Model file for the job. Use its own axes, mm. Face numbers are marked on the shaded views. A direction names the side the tool comes from. Coordinates: 2 decimals unless noted, no trailing zeros. Order: outer loops, then holes, each group sorted by start corner. A loop starts at its lowest first (then second) coordinate and runs counter-clockwise, first axis right, second up.
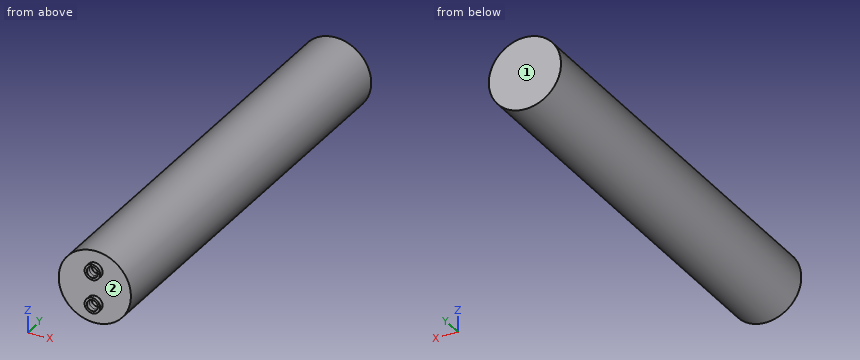
from build123d import *

# Parameters (mm, degrees)
F0_R     = 6.5
F1_DEPTH = 79
F2_T     = -0.8
F3_DEPTH = 0.8
F4_DEPTH = 0.8


with BuildPart() as f1:
    # F0 (on Front) → F1 (new body)
    with BuildSketch(Plane.XZ):
        with Locations((6.5, 6.5)):
            Circle(F0_R)
        with BuildLine():
            ThreePointArc((7.9, 3.5), (5.5100505063, 2.5100505063), (6.5, 4.9))
            ThreePointArc((6.5, 4.9), (7.4899494937, 4.4899494937), (7.9, 3.5))
        make_face(mode=Mode.SUBTRACT)
        with BuildLine():
            ThreePointArc((6.5, 8.1), (5.5100505063, 10.4899494937), (7.9, 9.5))
            ThreePointArc((7.9, 9.5), (7.4899494937, 8.5100505063), (6.5, 8.1))
        make_face(mode=Mode.SUBTRACT)
        with BuildLine():
            ThreePointArc((6.5, 8.1), (7.4899494937, 8.5100505063), (7.9, 9.5))
            ThreePointArc((7.9, 9.5), (5.5100505063, 10.4899494937), (6.5, 8.1))
        make_face()
        with BuildLine():
            ThreePointArc((7.5, 9.5), (7.2071067812, 8.7928932188), (6.5, 8.5))
            ThreePointArc((6.5, 8.5), (5.7928932188, 10.2071067812), (7.5, 9.5))
        make_face(mode=Mode.SUBTRACT)
        with BuildLine():
            ThreePointArc((7.9, 3.5), (7.4899494937, 4.4899494937), (6.5, 4.9))
            ThreePointArc((6.5, 4.9), (5.5100505063, 2.5100505063), (7.9, 3.5))
        make_face()
        with BuildLine():
            ThreePointArc((7.5, 3.5), (5.7928932188, 2.7928932188), (6.5, 4.5))
            ThreePointArc((6.5, 4.5), (7.2071067812, 4.2071067812), (7.5, 3.5))
        make_face(mode=Mode.SUBTRACT)
        with BuildLine():
            ThreePointArc((7.5, 9.5), (5.7928932188, 10.2071067812), (6.5, 8.5))
            ThreePointArc((6.5, 8.5), (7.2071067812, 8.7928932188), (7.5, 9.5))
        make_face()
        with BuildLine():
            ThreePointArc((7.5, 3.5), (7.2071067812, 4.2071067812), (6.5, 4.5))
            ThreePointArc((6.5, 4.5), (5.7928932188, 2.7928932188), (7.5, 3.5))
        make_face()
    extrude(amount=-F1_DEPTH)

    # F2
    f2_openings = [f1.faces().sort_by_distance(p)[0] for p in [
        (6.5, 0, 6.5),
    ]]
    offset(amount=F2_T, openings=f2_openings)

    # F0 (on Front) → F3 (join)
    with BuildSketch(Plane.XZ):
        with Locations((6.5, 6.5)):
            Circle(F0_R)
        with BuildLine():
            ThreePointArc((7.9, 3.5), (5.5100505063, 2.5100505063), (6.5, 4.9))
            ThreePointArc((6.5, 4.9), (7.4899494937, 4.4899494937), (7.9, 3.5))
        make_face(mode=Mode.SUBTRACT)
        with BuildLine():
            ThreePointArc((6.5, 8.1), (5.5100505063, 10.4899494937), (7.9, 9.5))
            ThreePointArc((7.9, 9.5), (7.4899494937, 8.5100505063), (6.5, 8.1))
        make_face(mode=Mode.SUBTRACT)
    extrude(amount=-F3_DEPTH)

    # F0 (on Front) → F4 (join, symmetric)
    with BuildSketch(Plane.XZ):
        with BuildLine():
            ThreePointArc((6.5, 8.1), (7.4899494937, 8.5100505063), (7.9, 9.5))
            ThreePointArc((7.9, 9.5), (5.5100505063, 10.4899494937), (6.5, 8.1))
        make_face()
        with BuildLine():
            ThreePointArc((7.5, 9.5), (7.2071067812, 8.7928932188), (6.5, 8.5))
            ThreePointArc((6.5, 8.5), (5.7928932188, 10.2071067812), (7.5, 9.5))
        make_face(mode=Mode.SUBTRACT)
        with BuildLine():
            ThreePointArc((7.9, 3.5), (7.4899494937, 4.4899494937), (6.5, 4.9))
            ThreePointArc((6.5, 4.9), (5.5100505063, 2.5100505063), (7.9, 3.5))
        make_face()
        with BuildLine():
            ThreePointArc((7.5, 3.5), (5.7928932188, 2.7928932188), (6.5, 4.5))
            ThreePointArc((6.5, 4.5), (7.2071067812, 4.2071067812), (7.5, 3.5))
        make_face(mode=Mode.SUBTRACT)
    extrude(amount=F4_DEPTH, both=True)


solid = f1.part
Q1. Cut at B-B, the plane x = 9.75. List the corners of the cut face in (y, z), plus the area to 3 significant figures.
Established:
outline: (0, 0.87) - (79, 0.87) - (79, 12.13) - (0, 12.13) - close; hole (0.8, 1.82) - (78.2, 1.82) - (78.2, 11.18) - (0.8, 11.18) - close
area: 165 mm2
Q2. Probe line 1 (Z direction, x = 6.5, y = -0.4); line 2 (Z direction, x = 6.5, y = 0.5); line 3 (X direction, y = -0.3, z = 3.5). List the from-to ranges inside material, lowest first.
Established:
line 1: z = 2.1 to 2.5, 4.5 to 4.9, 8.1 to 8.5, 10.5 to 10.9
line 2: z = 0 to 2.5, 4.5 to 8.5, 10.5 to 13
line 3: x = 5.1 to 5.5, 7.5 to 7.9
Q3. Cut at A-A, the plane z = 6.5. List the corners of the cut face in (x, y), plus the area to 3 significant figures.
Established:
outline: (0, 0) - (13, 0) - (13, 79) - (0, 79) - close; hole (0.8, 0.8) - (12.2, 0.8) - (12.2, 78.2) - (0.8, 78.2) - close
area: 145 mm2
Q4. Which spindle directions (+Z, -Z, +X, -X, +Y, -Y) get a long thin tool onto all of the face, cutting with end or side? Do the marked faces 1 and 2. Say none if no direction does.
Established:
face 1: +Z, -Z, +X, -X, +Y
face 2: -Y
Q5. Cut at C-C, the plane y = 9. List the corners of the cut face in (x, z), plus the area to 3 significant figures.
Established:
outline: circle Ø13 at (6.5, 6.5); hole circle Ø11.4 at (6.5, 6.5)
area: 30.7 mm2
Q6. Drop flat-ended pins along their axis: P1, Ø4, axis at x = 4.5, z = 6.5, coming from the -Y side; P2, Ø3, axis at x = 5.5, y = 28.5, coming from the +Z side; P3, Ø1.6, axis at x = 6.5, z = 9.5, coming from the -Y side; P4, Ø1.5, axis at y = 31, z = 8, coming from the -X side. Give the stop position or say it passes through.
Established:
P1: stops at y = 0
P2: stops at z = 13
P3: stops at y = 78.2
P4: stops at x = 0.04
